CAD build for the part. Positions are in the model's coordinates, mm. A direction names the side the tool comes from. Coordinates: 2 decimals unless noted, no trailing zeros. Loops run counter-clockwise (first coordinate to the right, second up) from the corner with the lowest first, then second, coordinate; pieces in that order, holes last. Notation, with made-up numbers: (34, 28.5) -> (52, 28.5) arc R24 cw to (52, 42.5) -> close; hole circle Ø11 at (-15, -0.75). An arc over 180 degrees is marked (long way). Answer as CSV lines item,"result". Start each with the question number.
```python
from build123d import *

# Parameters (mm, degrees)
ESQUISSE1_R             = 10
BOSS_EXTRU_1_DEPTH      = 15
BOSS_EXTRU_1_TAPER      = 2
CONG_1_R                = 5
ESQUISSE2_R             = 3
ENL_V_MAT_EXTRU_1_DEPTH = 12
ESQUISSE3_R             = 7.5
ENL_V_MAT_EXTRU_2_DEPTH = 5


with BuildPart() as part:
    # Esquisse1 → Boss.-Extru.1 (new body)
    with BuildSketch(Plane.XY):
        Circle(ESQUISSE1_R)
    extrude(amount=BOSS_EXTRU_1_DEPTH, taper=BOSS_EXTRU_1_TAPER)

    # Congé1
    cong_1_edges = [part.edges().sort_by_distance(p)[0] for p in [
        (-9.476188458, 0, 15),
    ]]
    fillet(cong_1_edges, radius=CONG_1_R)

    # Esquisse2 → Enlèv. mat.-Extru.1 (cut)
    with BuildSketch(Plane(origin=(0, 0, 0), x_dir=(-1, 0, 0), z_dir=(0, 0, -1))):
        Circle(ESQUISSE2_R)
    extrude(amount=-ENL_V_MAT_EXTRU_1_DEPTH, mode=Mode.SUBTRACT)

    # Esquisse3 → Enlèv. mat.-Extru.2 (cut)
    with BuildSketch(Plane(origin=(0, 0, 0), x_dir=(-1, 0, 0), z_dir=(0, 0, -1))):
        Circle(ESQUISSE3_R)
    extrude(amount=-ENL_V_MAT_EXTRU_2_DEPTH, mode=Mode.SUBTRACT)


solid = part.part
```
Q1. Which spindle directions (+Z, -Z, +X, -X, +Y, -Y) get a long thin tool onto all of the face, cutting with end or side? Do faces 1 (the flat face through (4, 7, 0)), 2 (the cylindrical face through (7.493, 0.33, 2.465)). Say none if no direction does.
Q2. Probe probe 1 along Z at (x, y) = (1.25, -3.25); probe 2 along Y at (x, z) = (0.25, 5.25); probe 3 along Y at (x, z) = (0, 2.3). List the from-to ranges inside material, lowest first. Write a range as from..to.
Q3. Pin check, flat tips, straight feed: pin 1 Ø8 at (y, z) = (7.5, 12) entering from -X; pin 2 Ø3 at (x, z) = (-4.5, 7) entering from -Y; pin 3 Ø3 at (x, z) = (-0.5, 2) entering from +Y; pin 4 Ø6 at (x, y) = (5, 4) entering from +Z. Stop position of each tip, or through.
Q4. Saw through at B-B (z = 6.5). List the corners of the cut face in (x, y), and give its area (3 significant figures).
Q5. Two-plate mould, pull along X, no slides. Class faces 3 (the conical face through (-2.129, -9.586, 5.158)), 4 (the flat face through (0, 0, 15)), 5 (the flat face through (-3.2, 0.1, 5)): pulls with the +X half, pulls with the -X half, needs draft (parallel to the pull), parting line crosses it, or undercut.
Q6. Saw through at A-A (z = 2.75). List the corners of the cut face in (x, y).
Ans:
1,face 1,"-Z, +X, -X, +Y, -Y"
1,face 2,"-Z"
2,probe 1,"z = 5..15"
2,probe 2,"y = -9.81..-2.99, 2.99..9.81"
2,probe 3,"y = -9.92..-7.5, 7.5..9.92"
3,pin 1,"stops at x = -8.85"
3,pin 2,"stops at y = -9.29"
3,pin 3,"stops at y = 9.98"
3,pin 4,"stops at z = 15"
4,outline,"circle Ø19.55 at (0, 0); hole circle Ø6 at (0, 0)"
4,area,"272 mm²"
5,face 3,"parting line crosses it"
5,face 4,"needs draft"
5,face 5,"undercut"
6,outline,"circle Ø19.81 at (0, 0); hole circle Ø15 at (0, 0)"
